Design review of the part built by this model. Coordinates are the model's own, in mm. Face numbers are marked on the shaded views. A direction names the side the tool comes from. Give positions to 0.01 mm unless a question says otherwise; leave off trailing zeros. Loops run counter-clockwise (first coordinate to the right, second up) from the corner with the lowest first, then second, coordinate; pieces in that order, holes last.
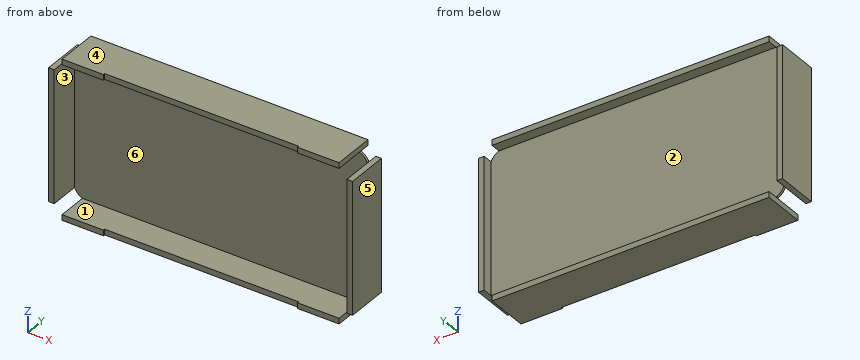
from build123d import *

# Parameters (mm, degrees)
SKETCH1_W             = 12.5
SKETCH1_H             = 293.5
BOSS_EXTRUDE1_DEPTH   = 93.8
SKETCH1_W_2           = 615.95
SKETCH1_H_2           = 12.5
BOSS_EXTRUDE1_2_DEPTH = 93.8
BOSS_EXTRUDE1_3_DEPTH = 93.8
BOSS_EXTRUDE1_4_DEPTH = 93.8
SKETCH2_W             = 650.95
SKETCH2_H             = 328.5
BOSS_EXTRUDE2_DEPTH   = 5
FILLET2_R             = 30
SKETCH4_W             = 215.725
SKETCH4_H             = 3.8
CUT_EXTRUDE1_DEPTH    = 498.983725261


with BuildPart() as part:
    # Sketch1 → Boss-Extrude1 (new body)
    with BuildSketch(Plane(origin=(0, 0, 0), x_dir=(1, 0, 0), z_dir=(0, 1, 0))):
        with Locations((-331.725, 0)):
            Rectangle(SKETCH1_W, SKETCH1_H)
    extrude(amount=BOSS_EXTRUDE1_DEPTH)



with BuildPart() as body_2:
    # Sketch1 → Boss-Extrude1 2 (new body)
    with BuildSketch(Plane(origin=(0, 0, 0), x_dir=(1, 0, 0), z_dir=(0, 1, 0))):
        with Locations((0, 170.5)):
            Rectangle(SKETCH1_W_2, SKETCH1_H_2)
    extrude(amount=BOSS_EXTRUDE1_2_DEPTH)


with BuildPart() as body_3:
    # Sketch1 → Boss-Extrude1 3 (new body)
    with BuildSketch(Plane(origin=(0, 0, 0), x_dir=(1, 0, 0), z_dir=(0, 1, 0))):
        with Locations((331.725, 0)):
            Rectangle(SKETCH1_W, SKETCH1_H)
    extrude(amount=BOSS_EXTRUDE1_3_DEPTH)


with BuildPart() as body_4:
    # Sketch1 → Boss-Extrude1 4 (new body)
    with BuildSketch(Plane(origin=(0, 0, 0), x_dir=(1, 0, 0), z_dir=(0, 1, 0))):
        with Locations((0, -170.5)):
            Rectangle(SKETCH1_W_2, SKETCH1_H_2)
    extrude(amount=BOSS_EXTRUDE1_4_DEPTH)


with BuildPart() as part_1:
    add(part.part)

    add(body_2.part)  # Boss-Extrude2 merges body 2

    add(body_3.part)  # Boss-Extrude2 merges body 3

    add(body_4.part)  # Boss-Extrude2 merges body 4
    # Sketch2 → Boss-Extrude2 (add)
    with BuildSketch(Plane(origin=(0, 71.25, 0), x_dir=(1, 0, 0), z_dir=(0, 1, 0))):
        Rectangle(SKETCH2_W, SKETCH2_H)
    extrude(amount=-BOSS_EXTRUDE2_DEPTH)

    # Fillet2
    # the kernel refuses this fillet: 30 mm, written as the material it takes off along each edge
    with BuildSketch(Plane(origin=(-325.475, 115, 164.25), x_dir=(1, 0, 0), z_dir=(0, -1, 0)), Plane(origin=(-325.475, 115, -164.25), x_dir=(0, 0, 1), z_dir=(0, -1, 0)), Plane(origin=(325.475, 115, -164.25), x_dir=(-1, 0, 0), z_dir=(0, -1, 0)), Plane(origin=(325.475, 115, 164.25), x_dir=(0, 0, -1), z_dir=(0, -1, 0))) as fillet2_piece_1:
        with BuildLine():
            CenterArc((28.074531042, -28.074531042), FILLET2_R, 110.63934566, 48.721308679)
            Line((0, -17.5), (0, 0))
            Line((0, 0), (17.5, 0))
        make_face()
    extrude(amount=92.5, mode=Mode.SUBTRACT)

    # Sketch4 → Cut-Extrude1 (cut, through all)
    with BuildSketch(Plane(origin=(0, 0, -176.75), x_dir=(-1, 0, 0), z_dir=(0, 0, -1))):
        with Locations((-107.8625, 1.9)):
            Rectangle(SKETCH4_W, SKETCH4_H)
        with Locations((107.8625, 1.9)):
            Rectangle(SKETCH4_W, SKETCH4_H)
    extrude(amount=-CUT_EXTRUDE1_DEPTH, mode=Mode.SUBTRACT)


solid = part_1.part
Q1. Take a section at A-A (y = 17.5). Give the boundary of the cut face in (x, z) (3 decimals), plus the area to 3 significant figures.
Results:
outline: (-337.975, -146.75) - (-325.475, -146.75) - (-325.475, 146.75) - (-337.975, 146.75) - close; (-307.975, -176.75) - (307.975, -176.75) - (307.975, -164.25) - (-307.975, -164.25) - close; (-307.975, 164.25) - (307.975, 164.25) - (307.975, 176.75) - (-307.975, 176.75) - close; (325.475, -146.75) - (337.975, -146.75) - (337.975, 146.75) - (325.475, 146.75) - close
area: 22,700 mm2
Q2. Draft analysis for pull direction Z (two halves, no side actions). For the marked faces 1, 2, 3 and 4, state which applies: pulls with the +Z half, pulls with the -Z half, needs draft (parallel to the pull), parting line crosses it, or undercut.
Results:
face 1: undercut
face 2: undercut
face 3: needs draft
face 4: pulls with the +Z half
Q3. Take a section at B-B (z = -46). Give the boundary of the cut face in (x, y) (3 decimals).
Results:
outline: (-337.975, 0) - (-325.475, 0) - (-325.475, 66.25) - (325.475, 66.25) - (325.475, 0) - (337.975, 0) - (337.975, 93.8) - (325.475, 93.8) - (325.475, 71.25) - (-325.475, 71.25) - (-325.475, 93.8) - (-337.975, 93.8) - close
Q4. Take a section at C-C (x = 246). Give the boundary of the cut face in (y, z), plus the area to 3 significant figures.
Results:
outline: (0, -176.75) - (93.8, -176.75) - (93.8, -164.25) - (71.25, -164.25) - (71.25, 164.25) - (93.8, 164.25) - (93.8, 176.75) - (0, 176.75) - (0, 164.25) - (66.25, 164.25) - (66.25, -164.25) - (0, -164.25) - close
area: 3,990 mm2
Q5. Tool access review of the marked faces 5 and 6: name each direction out of +Z, -Z, +X, -X, +Y, -Y from which nothing blocks a thin tool from reaching the whole face with its end or side.
Results:
face 5: +Z, -Z, +X, +Y, -Y
face 6: -Y
Q6. Insertion check: pin 1 (3 mm diameter, centred on y = 1, z = -169.5, fed in from +X) (3 decimals); pin 2 (6 mm diameter, centred on x = 59, z = 167.5, fed in from -Y); pin 3 (10 mm diameter, centred on x = 147.5, z = 32, fed in from -Y). Each pin has a flat end and moves straight along its axis. Give the tip position at first contact, or say it passes through.
Results:
pin 1: stops at x = 307.975
pin 2: stops at y = 3.8
pin 3: stops at y = 66.25
Q7. Wall thickness on line 1 (X direction, y = 64, z = -121.5) (3 decimals); line 2 (Z direction, x = 182.5, y = 20); line 3 (Y direction, x = 66.5, z = -126): over which ranges is each line inside the solid? List them lowest first.
Results:
line 1: x = -337.975 to -325.475, 325.475 to 337.975
line 2: z = -176.75 to -164.25, 164.25 to 176.75
line 3: y = 66.25 to 71.25
